```python
from build123d import *

# Parameters (mm, degrees)
SKETCH2_W           = 30
SKETCH2_H           = 30
BOSS_EXTRUDE2_DEPTH = 10
CUT_EXTRUDE2_DEPTH  = 36
SKETCH6_R           = 5
BOSS_EXTRUDE3_DEPTH = 15
SKETCH7_R           = 4.109940847
CUT_EXTRUDE3_DEPTH  = 2


with BuildPart() as part:
    # Sketch2 → Boss-Extrude2 (new body)
    with BuildSketch(Plane.XY):
        Rectangle(SKETCH2_W, SKETCH2_H)
    extrude(amount=BOSS_EXTRUDE2_DEPTH)

    # Sketch5 → Cut-Extrude2 (cut)
    with BuildSketch(Plane(origin=(15, 0, 0), x_dir=(0, 0, -1), z_dir=(1, 0, 0))):
        Polygon((0, 15), (-10, -1.73373583), (-10, 15), align=None)
    extrude(amount=-CUT_EXTRUDE2_DEPTH, mode=Mode.SUBTRACT)

    # Sketch6 → Boss-Extrude3 (add)
    with BuildSketch(Plane(origin=(0, 3.947182334, 6.605110645), x_dir=(1, 0, 0), z_dir=(0, 0.512977084, 0.858402301))):
        Circle(SKETCH6_R)
    extrude(amount=BOSS_EXTRUDE3_DEPTH)

    # Sketch7 → Cut-Extrude3 (cut)
    with BuildSketch(Plane(origin=(0, 11.641838597, 19.481145166), x_dir=(1, 0, 0), z_dir=(0, 0.512977084, 0.858402301))):
        Circle(SKETCH7_R)
    extrude(amount=-CUT_EXTRUDE3_DEPTH, mode=Mode.SUBTRACT)


solid = part.part
```
For this review, take the finished solid that the model builds, in its own axes (mm). A direction names the side the tool comes from. Coordinates: 2 decimals unless noted, no trailing zeros. Write each loop counter-clockwise with the first axis right and the second up, starting at its lowest first coordinate (ties: lowest second). Pieces come first, ordered by that corner, then holes.
(1) Tool access review of faces 4 (the face through (-0.06, 10.67, 17.73)), 5 (the face through (0, -8, 10)), 6 (the face through (0, 0, 0)): name each direction out of +Z, -Z, +X, -X, +Y, -Y from which nothing blocks a thin tool from reaching the whole face with its end or side.
(2) Wall thickness on probe 1 along Z at (x, y) = (-10, -10); probe 2 along X at (y, z) = (6, 10); probe 3 along Z at (x, y) = (-8, 3): over which ranges is each line inside the solid? List them lowest first.
(3) Add section A-A on y = -4.5. Give the boundary of the cut face in (x, z), then the cut area to 3 significant figures.
(4) The part is to be moulded in two halves that separate along Y. For faces 1 (the face through (0, -15, 5)), 2 (the face through (-15, -4, 4)), 3 (the face through (3.92, 12.2, 18)), say which applies: +Y half, -Y half, draft (parallel to the pull), parting line (faces both ways), or undercut.
(5) For pin 1 Ø10 at (x, z) = (3.5, 12.5) entering from +Y; pin 2 Ø1.5 at (y, z) = (10, 5) entering from +X; pin 3 Ø4 at (x, z) = (0.5, 4) entering from +Y; pin 4 Ø4 at (x, z) = (-1.5, 14) entering from -Y, all flat-tipped, find the tip position at first contact; note any pin that passes through.
(6) Add section B-B on x = 8. Give the boundary of the cut face in (y, z).
Answer sheet:
1. face 4: none
1. face 5: +Z, +X, -X, -Y
1. face 6: -Z, +X, -X, +Y, -Y
2. probe 1: z = 0 to 10
2. probe 2: x = -5 to 5
2. probe 3: z = 0 to 7.17
3. outline: (-15, 0) - (15, 0) - (15, 10) - (-15, 10) - close
3. area: 300 mm2
4. face 1: -Y half
4. face 2: draft
4. face 3: undercut
5. pin 1: stops at y = 15.78
5. pin 2: passes through
5. pin 3: stops at y = 11.65
5. pin 4: stops at y = 1.5
6. outline: (-15, 0) - (15, 0) - (-1.73, 10) - (-15, 10) - close
